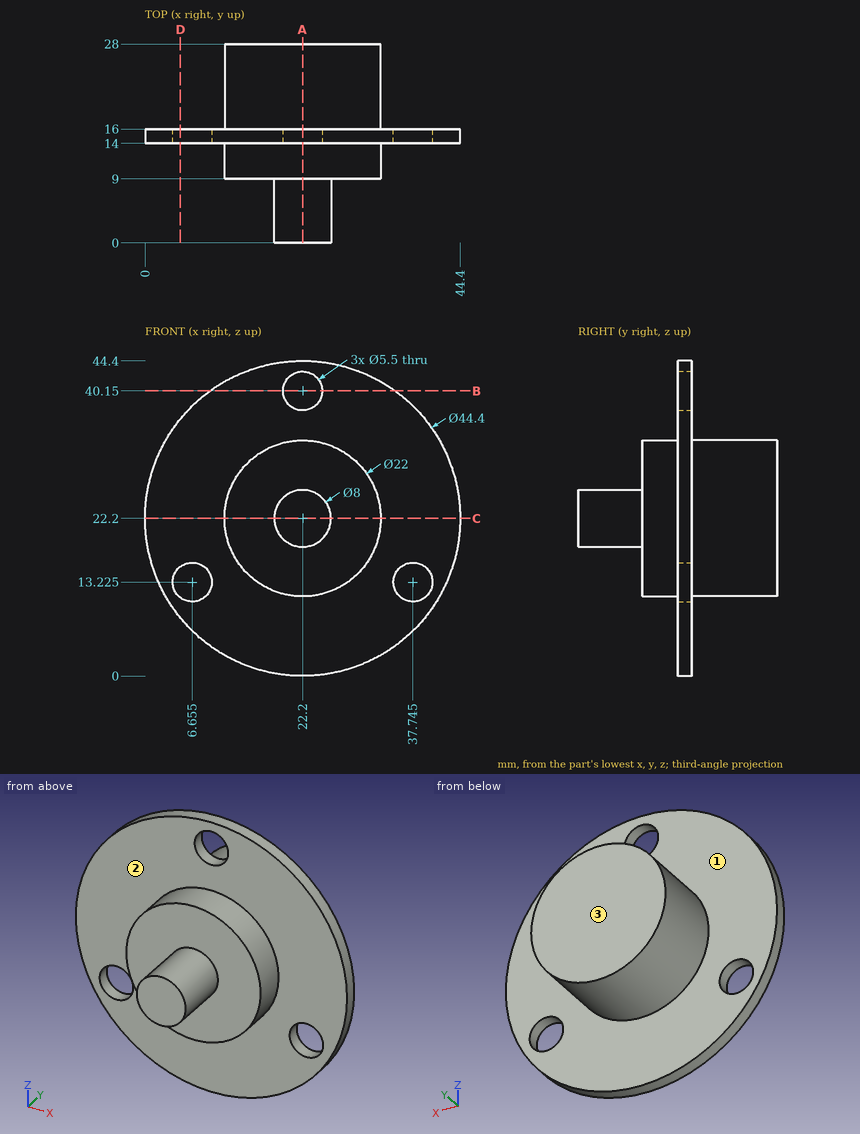
Verification items for this drawing (mm, ordinates from the low corner). A direction names the side the tool comes from. Round coordinates to 2 decimals unless told otherwise and drop trailing zeros. Order: outer loops, then holes, each group sorted by start corner. A loop starts at its lowest first (then second) coordinate and runs counter-clockwise, first axis right, second up.
1) Tool access check on the marked faces 1, 2 and 3. Record the directions out of +Z, -Z, +X, -X, +Y, -Y that give a thin tool (end or side, any length) a straight path to the whole face; none if there is none.
Geometry says:
face 1: +Y
face 2: -Y
face 3: +Z, -Z, +X, -X, +Y
2) Cross-section at C-C, the plane z = 22.2. Record the cut outline in (x, y).
Geometry says:
outline: (0, 14) - (11.2, 14) - (11.2, 9) - (18.2, 9) - (18.2, 0) - (26.2, 0) - (26.2, 9) - (33.2, 9) - (33.2, 14) - (44.4, 14) - (44.4, 16) - (33.2, 16) - (33.2, 28) - (11.2, 28) - (11.2, 16) - (0, 16) - close
3) Material ranges on line 1 (Y direction, x = 32, z = 41); line 2 (Y direction, x = 23.5, z = 14.5); line 3 (X direction, y = 14.9, z = 40.15), recorded low to high.
Geometry says:
line 1: y = 14 to 16
line 2: y = 9 to 28
line 3: x = 9.14 to 19.45, 24.95 to 35.26
4) Depth check by flat-ended pin: pin 1 (5 mm diameter, centred on y = 21, z = 21.5, fed in from -X); pin 2 (5 mm diameter, centred on x = 39.5, y = 16.5, fed in from -Z); pin 3 (6 mm diameter, centred on y = 16, z = 12, fed in from -X); pin 4 (6 mm diameter, centred on y = 22, z = 6.5, fed in from -X). Enter the tip coordinate at first touch or a pass-through.
Geometry says:
pin 1: stops at x = 11.2
pin 2: stops at z = 5.7
pin 3: stops at x = 1.2
pin 4: passes through
5) Cross-section at B-B, the plane z = 40.15. Record the cut outline in (x, y).
Geometry says:
outline: (9.14, 14) - (19.45, 14) - (19.45, 16) - (9.14, 16) - close; (24.95, 14) - (35.26, 14) - (35.26, 16) - (24.95, 16) - close
6) Cross-section at A-A, the plane x = 22.2. Record the cut outline in (y, z), plus the area to 3 significant figures.
Geometry says:
outline: (0, 18.2) - (9, 18.2) - (9, 11.2) - (14, 11.2) - (14, 0) - (16, 0) - (16, 11.2) - (28, 11.2) - (28, 33.2) - (16, 33.2) - (16, 37.4) - (14, 37.4) - (14, 33.2) - (9, 33.2) - (9, 26.2) - (0, 26.2) - close; (14, 42.9) - (16, 42.9) - (16, 44.4) - (14, 44.4) - close
area: 524 mm2
7) Cross-section at D-D, the plane x = 5. Record the cut outline in (y, z).
Geometry says:
outline: (14, 8.16) - (16, 8.16) - (16, 11.03) - (14, 11.03) - close; (14, 15.42) - (16, 15.42) - (16, 36.24) - (14, 36.24) - close
